Autodesk Inventor part; units mm, degrees
ref_plane "YZ Plane" through (0, 0, 0) normal (1, 0, 0) x (0, 1, 0)
ref_plane "XZ Plane" through (0, 0, 0) normal (0, 1, 0) x (-1, 0, 0)
ref_plane "XY Plane" through (0, 0, 0) normal (0, 0, 1) x (1, 0, 0)
sketch "Sketch1" plane through (0, 0, 0) normal (0, 1, 0) x (-1, 0, 0)
  line L0 (100, 0) -> (0, 0)
  line L1 (0, 0) -> (0, -100)
  line L2 (0, -100) -> (100, -100)
  line L3 (100, -100) -> (100, 0)
  dimension "d0" = 100
extrude "Extrusion1" add sketch "Sketch1" along normal blind 10
sketch "Sketch2" plane through (0, 10, 0) normal (0, 1, 0) x (1, 0, 0)
  line L0 (-20, 20) -> (-80, 20) construction
  line L1 (-80, 20) -> (-80, 80) construction
  line L2 (-80, 80) -> (-20, 80) construction
  line L3 (-20, 80) -> (-20, 20) construction
  line L4 (-100, 0) -> (0, 0) construction
  line L5 (0, 0) -> (0, 100) construction
  dimension "d3" = 60
  dimension "d4" = 20
  dimension "d5" = 20
hole "Hole1" at (-20, 10, -20) at (-80, 10, -20) at (-20, 10, -80) at (-80, 10, -80) direction (0, -1, 0) diameter 6.3 depth 7.5 tip angle 118
sketch "Sketch3" plane through (0, 10, 0) normal (0, 1, 0) x (1, 0, 0)
  circle A0 centre (-80, 20) radius 3.15
  circle A1 centre (-20, 20) radius 3.15
  circle A2 centre (-80, 80) radius 3.15
  circle A3 centre (-20, 80) radius 3.15
  point P0 (0, 0)
hole "Hole2" at (-80, 10, -20) at (-20, 10, -20) at (-80, 10, -80) at (-20, 10, -80) direction (0, -1, 0) diameter 10.8 depth 5 tip angle 118
fillet "Fillet1" radius 2 4 edges at (-100, 5, 0) (0, 5, 0) (0, 5, -100) (-100, 5, -100)
sketch "Sketch4" plane through (0, 0, 0) normal (0, -1, 0) x (1, 0, 0)
  line L0 (60, -37.5) -> (0, -37.5)
  line L1 (0, -37.5) -> (0, -62.5)
  line L2 (0, -62.5) -> (60, -62.5)
  line L3 (60, -62.5) -> (60, -37.5)
  line L4 (0, -2) -> (0, -98)
  line L5 (60, -50) -> (0, -50) construction
  line L6 (-98, 0) -> (-2, 0) construction
  point P0 (0, 0)
  dimension "d21" = 25
  dimension "d22" = 60
  dimension "d23" = 50
extrude "Extrusion2" add sketch "Sketch4" against normal blind 3
fillet "Fillet2" radius 2 4 edges at (0, 1.5, -37.5) (60, 1.5, -37.5) (60, 1.5, -62.5) (0, 1.5, -62.5)
equation "\"d0\" = base_width"
equation "\"d1\" = base_thickness"
equation "\"d3\" = rod_dist"
equation "\"d4\" = 0.5 * base_width - 0.5 * rod_dist"
equation "\"d5\" = 0.5 * base_width - 0.5 * rod_dist"
equation "\"d6\" = rod_tolerance + rod_diameter"
equation "\"d11\" = 0.75 * base_thickness"
equation "\"d13\" = rod_tolerance + post_diameter"
equation "\"d18\" = 0.5 * base_thickness"
equation "\"d21\" = flange_width"
equation "\"d22\" = flange_length"
equation "\"d23\" = 0.5 * base_width"
equation "\"base_width\" = 100"
equation "\"base_thickness\" = 10"
equation "\"rod_diameter\" = 6"
equation "\"rod_tolerance\" = 0.3"
equation "\"flange_length\" = 60"
equation "\"flange_width\" = 25"
equation "\"post_diameter\" = 10.5"
equation "\"rod_dist\" = 60"
properties part number "cradle_base"
Model file for the job. Use its own axes, mm. A direction names the side the tool comes from. Round coordinates to 2 decimals unless told otherwise and drop trailing zeros. Order: outer loops, then holes, each group sorted by start corner. A loop starts at its lowest first (then second) coordinate and runs counter-clockwise, first axis right, second up. Notation, with made-up numbers: M -0.75,43 L 12.25,43 A19 cw 12.25,68 Z; hole C 44.5,-11.5 d11. An arc over 180 degrees is marked long. Use CSV: the item, a comma, the result in double quotes.
Item 1: Saw through at A-A (y = 7). List the corners of the cut face in (x, z), plus the area to 3 significant figures.
Worked answers:
outline,"M -100,-98 A2 ccw -98,-100 L -2,-100 A2 ccw 0,-98 L 0,-2 A2 ccw -2,0 L -98,0 A2 ccw -100,-2 Z; hole C -80,-80 d10.8; hole C -80,-20 d10.8; hole C -20,-80 d10.8; hole C -20,-20 d10.8"
area,"9,630 mm²"
Item 2: Pull direction X, two halves, no side cores. Call faces 4 (the face through (0, 5, -49)), 5 (the face through (-100, 5, -51)), 6 (the face through (-19.012, 3.733, -76.861)): released by +X, released by -X, zero draft, split by the parting line, or undercut.
Worked answers:
face 4,"released by +X"
face 5,"released by -X"
face 6,"undercut"
Item 3: Pin check, flat tips, straight feed: pin 1 (6 mm diameter, centred on x = 26.5, y = 1, fed in from -Z); pin 2 (8 mm diameter, centred on x = -80, z = -80, fed in from +Y); pin 3 (3 mm diameter, centred on y = 4, z = -29.5, fed in from +X). Stop position of each tip, or through.
Worked answers:
pin 1,"z = -62.5"
pin 2,"y = 4.16"
pin 3,"x = 0"
Item 4: Which spindle directions (+Z, -Z, +X, -X, +Y, -Y) get a long thin tool onto all of the face, cutting with end or side? Do faces 1 (the face through (-51, 5, 0)), 2 (the face through (30, 3, -50)), 3 (the face through (-80.138, 3.066, -83.147)). Say none if no direction does.
Worked answers:
face 1,"+Z, +X, -X, +Y, -Y"
face 2,"+Z, -Z, +X, +Y"
face 3,"+Y"
Item 5: Saw through at C-C (x = 6.5). List the corners of the cut face in (y, z).
Worked answers:
outline,"M 0,-62.5 L 3,-62.5 L 3,-37.5 L 0,-37.5 Z"
Item 6: Probe probe 1 along X at (y, z) = (7.25, -20); probe 2 along X at (y, z) = (2.95, -20). List the from-to ranges inside material, lowest first.
Worked answers:
probe 1,"-100 to -85.4, -74.6 to -25.4, -14.6 to 0"
probe 2,"-100 to -83.15, -76.85 to -23.15, -16.85 to 0"
Item 7: Saw through at B-B (z = -46). List the corners of the cut face in (x, y), plus the area to 3 significant figures.
Worked answers:
outline,"M -100,0 L 60,0 L 60,3 L 0,3 L 0,10 L -100,10 Z"
area,"1,180 mm²"
